Source: CAD feature listing. Evaluate the final solid. Frame: model axes, mm. Coordinates: 2 decimals unless noted, no trailing zeros. Order: outer loops, then holes, each group sorted by start corner. A loop starts at its lowest first (then second) coordinate and runs counter-clockwise, first axis right, second up. Notation, with made-up numbers: (39.25, 85) -> (77.25, 85) arc R19 ccw to (77.25, 106) -> close; hole circle Ø8 at (-20.5, 63.5). An arc over 180 degrees is marked (long way). Write item = value, one per line. Start each with the question number.
Item 1: Contact query for flat-ended pins moving along their axis: pin 1 (4 mm diameter, centred on x = -79.5, y = 2, fed in from +Z); pin 2 (5 mm diameter, centred on x = -40.5, z = -37.5, fed in from -Y); pin 3 (9 mm diameter, centred on x = -76.5, z = -8, fed in from +Y). Output: stop coordinate, or through.
Item 2: Section query B-B (x = 0). Output: boundary loops of the cut face in (y, z), then the cut area to 3 significant figures.
Item 3: Section query C-C (y = -8). Output: boundary loops of the cut face in (x, z).
Item 4: Section query A-A (z = -13.5). Output: boundary loops of the cut face in (x, y).
Item 5: Ray query, line 1 along Y through (x, z) = (0, -73); line 2 along X through (y, z) = (58, -65.5). Return the intervals inside material, ascending. Write a range as [from, to].
Item 6: Section query D-D (y = 69.5). Output: boundary loops of the cut face in (x, z), then the cut area to 3 significant figures.
```python
from build123d import *

# Parameters (mm, degrees)
SKETCH1_R               = 83.4771
SKETCH1_R_2             = 72.5043
BOSS_EXTRUDE1_DEPTH     = 65.0875
SKETCH3_W               = 101.6
SKETCH3_H               = 28.575
CUT_EXTRUDE2_DEPTH      = 84.4771
CUT_EXTRUDE2_DEPTH_BACK = 84.4771
SKETCH4_R               = 50.8
CUT_EXTRUDE3_DEPTH      = 98.7646
SKETCH6_W               = 101.6
SKETCH6_H               = 3.175
CUT_EXTRUDE4_DEPTH      = 84.4771001
CUT_EXTRUDE4_DEPTH_BACK = 84.4771001
SKETCH9_R               = 83.4771
SKETCH9_R_2             = 72.5043
BOSS_EXTRUDE2_DEPTH     = 508
SKETCH13_W              = 203.2
SKETCH13_H              = 2032
CUT_EXTRUDE7_DEPTH      = 762
SKETCH15_W              = 203.2
SKETCH15_H              = 203.2
CUT_EXTRUDE9_DEPTH      = 203.2
SKETCH16_R              = 83.4771
SKETCH16_R_2            = 72.5043
BOSS_EXTRUDE3_DEPTH     = 12.7


with BuildPart() as part:
    # Sketch1 → Boss-Extrude1 (new body, symmetric)
    with BuildSketch(Plane.XY):
        Circle(SKETCH1_R)
        Circle(SKETCH1_R_2, mode=Mode.SUBTRACT)
    extrude(amount=BOSS_EXTRUDE1_DEPTH, both=True)

    # Sketch3 → Cut-Extrude2 (cut, two sides)
    with BuildSketch(Plane(origin=(0, 0, 0), x_dir=(0, 0, -1), z_dir=(1, 0, 0))) as cut_extrude2_sk:
        with Locations((11.1125, 0)):
            Rectangle(SKETCH3_W, SKETCH3_H)
    extrude(amount=CUT_EXTRUDE2_DEPTH, mode=Mode.SUBTRACT)
    extrude(cut_extrude2_sk.sketch, amount=-CUT_EXTRUDE2_DEPTH_BACK, mode=Mode.SUBTRACT)

    # Sketch4 → Cut-Extrude3 (cut, through all)
    with BuildSketch(Plane(origin=(0, -14.2875, 0), x_dir=(1, 0, 0), z_dir=(0, 1, 0))):
        with Locations((-82.245325509, 11.1125)):
            Circle(SKETCH4_R)
        with Locations((82.245325509, 11.1125)):
            Circle(SKETCH4_R)
    extrude(amount=CUT_EXTRUDE3_DEPTH, mode=Mode.SUBTRACT)

    # Sketch6 → Cut-Extrude4 (cut, two sides)
    with BuildSketch(Plane(origin=(0, 0, 0), x_dir=(0, 0, -1), z_dir=(1, 0, 0))) as cut_extrude4_sk:
        with Locations((11.1125, 15.875)):
            Rectangle(SKETCH6_W, SKETCH6_H)
    extrude(amount=CUT_EXTRUDE4_DEPTH, mode=Mode.SUBTRACT)
    extrude(cut_extrude4_sk.sketch, amount=-CUT_EXTRUDE4_DEPTH_BACK, mode=Mode.SUBTRACT)

    # Sketch9 → Boss-Extrude2 (add)
    with BuildSketch(Plane.XY.offset(65.0875)):
        Circle(SKETCH9_R)
        Circle(SKETCH9_R_2, mode=Mode.SUBTRACT)
    extrude(amount=BOSS_EXTRUDE2_DEPTH)

    # Sketch13 → Cut-Extrude7 (cut)
    with BuildSketch(Plane(origin=(0, -43.994090512, 25.4), x_dir=(-1, 0, 0), z_dir=(0, 0.866025404, -0.5))):
        with Locations((0, 87.988181024)):
            Rectangle(SKETCH13_W, SKETCH13_H)
    extrude(amount=-CUT_EXTRUDE7_DEPTH, mode=Mode.SUBTRACT)

    # Sketch15 → Cut-Extrude9 (cut)
    with BuildSketch(Plane(origin=(0, 0, 177.4825), x_dir=(-1, 0, 0), z_dir=(0, 0, -1))):
        Rectangle(SKETCH15_W, SKETCH15_H)
    extrude(amount=-CUT_EXTRUDE9_DEPTH, mode=Mode.SUBTRACT)

    # Sketch16 → Boss-Extrude3 (add)
    with BuildSketch(Plane(origin=(0, 0, -65.0875), x_dir=(-1, 0, 0), z_dir=(0, 0, -1))):
        Circle(SKETCH16_R)
        Circle(SKETCH16_R_2, mode=Mode.SUBTRACT)
    extrude(amount=BOSS_EXTRUDE3_DEPTH)


solid = part.part
```
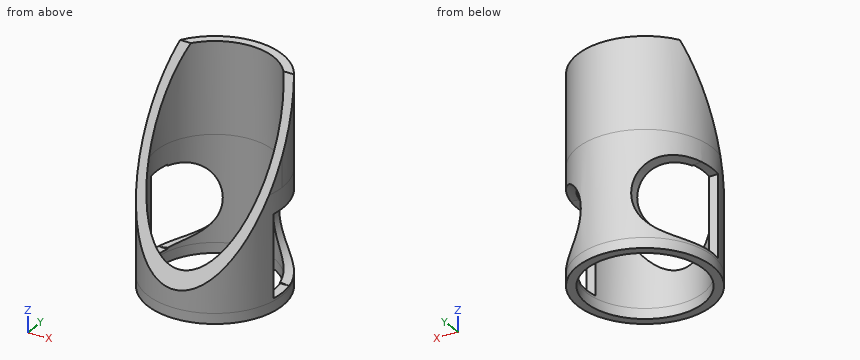
Computed:
q1.pin_1 = 108.53
q1.pin_2 = -74.33
q1.pin_3 = -14.29
q2.outline = (-83.48, -77.79) -> (-72.5, -77.79) -> (-72.5, -23.98) -> (-83.48, -42.99) -> close; (72.5, -77.79) -> (83.48, -77.79) -> (83.48, 177.48) -> (72.5, 177.48) -> close
q2.area = 3,290 mm^2
q3.outline = (-83.09, -77.79) -> (-72.06, -77.79) -> (-72.06, -61.91) -> (-83.09, -61.91) -> close; (-83.09, 39.69) -> (-72.06, 39.69) -> (-72.06, 87.74) -> (-83.09, 87.74) -> close; (72.06, -77.79) -> (83.09, -77.79) -> (83.09, -61.91) -> (72.06, -61.91) -> close; (72.06, 39.69) -> (83.09, 39.69) -> (83.09, 87.74) -> (72.06, 87.74) -> close
q4.outline = (-82.25, -14.29) arc R83.48 ccw to (-50.52, -66.45) -> (-29, -66.45) arc R72.5 cw to (-71.08, -14.29) -> close; (-31.5, 65.3) arc R72.5 cw to (31.5, 65.3) -> (31.5, 77.31) arc R83.48 ccw to (-31.5, 77.31) -> close; (29, -66.45) -> (50.52, -66.45) arc R83.48 ccw to (82.25, -14.29) -> (71.08, -14.29) arc R72.5 cw to start
q5.line_1 = [-83.48, -72.5], [72.5, 83.48]
q5.line_2 = [-60.04, -43.51], [43.51, 60.04]
q6.outline = (-46.24, -77.79) -> (-20.65, -77.79) -> (-20.65, 177.48) -> (-46.24, 177.48) -> (-46.24, 24.72) arc R50.8 cw to (-46.24, -46.95) -> close; (20.65, -77.79) -> (46.24, -77.79) -> (46.24, -46.95) arc R50.8 cw to (46.24, 24.72) -> (46.24, 177.48) -> (20.65, 177.48) -> close
q6.area = 11,600 mm^2
